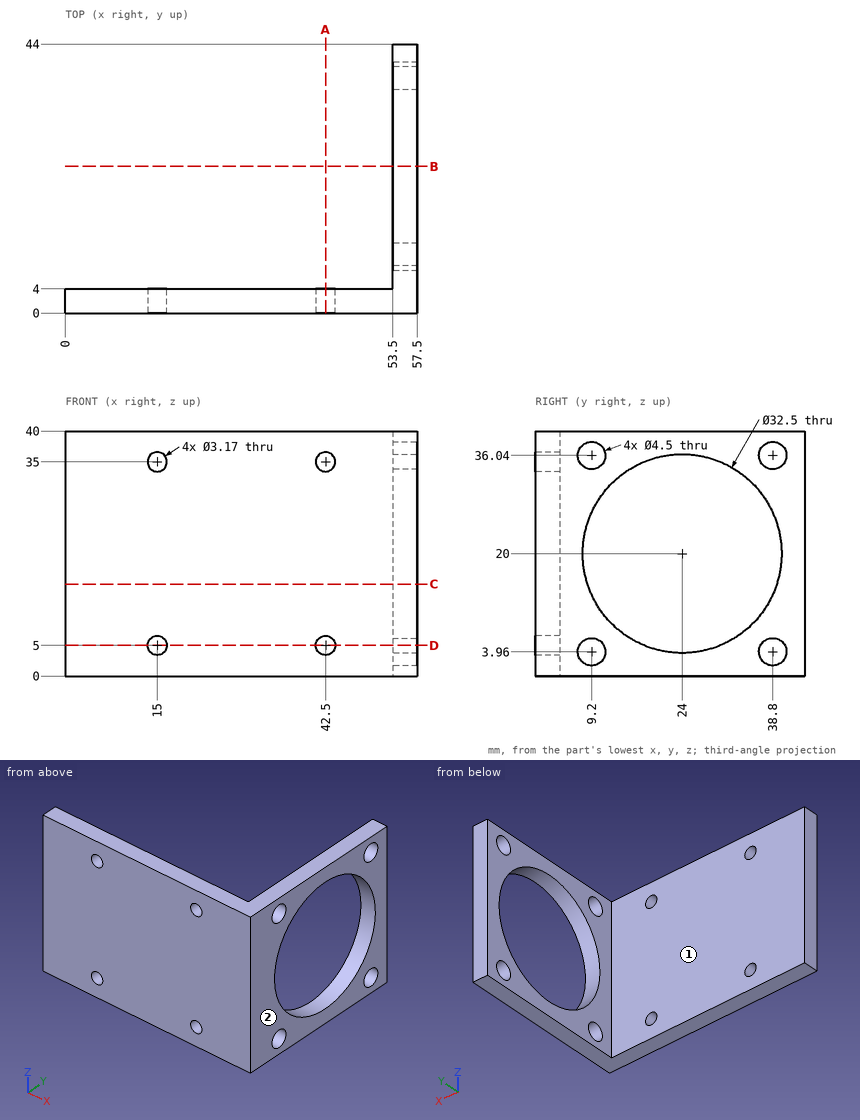
Print and shaded views of the part. All mm, measured from the part's lowest x, y and z. A direction names the side the tool comes from. Round coordinates to 2 decimals unless told otherwise and drop trailing zeros. Write each loop counter-clockwise with the first axis right and the second up, starting at its lowest first coordinate (ties: lowest second). Pieces come first, ordered by that corner, then holes. Notation, with made-up numbers: (-1, -10.5) -> (39, -10.5) arc R15 cw to (39, 1.5) -> close; hole circle Ø8 at (13, 17). An arc over 180 degrees is marked (long way). Answer in a Markdown table with one row per item. Add a question column.
Item 1: Which spindle directions (+Z, -Z, +X, -X, +Y, -Y) get a long thin tool onto all of the face, cutting with end or side? Do the marked faces 1 and 2. Say none if no direction does.
Item 2: Saw through at B-B, the plane y = 24. Write the cut outline in (x, z).
Item 3: Saw through at D-D, the plane z = 5. Write the cut outline in (x, y) (3 decimals), then the cut area to 3 significant figures.
Item 4: Drop flat-ended pins along their axis: pin 1 Ø12 at (x, z) = (17.5, 4) entering from +Y; pin 2 Ø5 at (y, z) = (9.2, 3.96) entering from -X. Give the stop position or say it passes through.
Item 5: Drill centre lines: line 1 (Z direction, x = 15, y = 3) (3 decimals); line 2 (X direction, y = 2.7, z = 5) (3 decimals); line 3 (Y direction, x = 54.5, z = 20). Where is each one in solid material? Low to high. Write a range as from..to.
Item 6: Saw through at A-A, the plane x = 42.5. Write the cut outline in (y, z) (3 decimals).
Item 7: Saw through at C-C, the plane z = 15. Write the cut outline in (x, y).
Findings below:
| question | item | result |
|---|---|---|
| 1 | face 1 | +Z, -Z, -X, +Y |
| 1 | face 2 | +Z, -Z, +X, +Y, -Y |
| 2 | outline | (53.5, 0) -> (57.5, 0) -> (57.5, 3.75) -> (53.5, 3.75) -> close; (53.5, 36.25) -> (57.5, 36.25) -> (57.5, 40) -> (53.5, 40) -> close |
| 3 | outline | (0, 0) -> (13.415, 0) -> (13.415, 4) -> (0, 4) -> close; (16.585, 0) -> (40.915, 0) -> (40.915, 4) -> (16.585, 4) -> close; (44.085, 0) -> (57.5, 0) -> (57.5, 7.205) -> (53.5, 7.205) -> (53.5, 4) -> (44.085, 4) -> close; (53.5, 11.195) -> (57.5, 11.195) -> (57.5, 17.75) -> (53.5, 17.75) -> close; (53.5, 30.25) -> (57.5, 30.25) -> (57.5, 36.805) -> (53.5, 36.805) -> close; (53.5, 40.795) -> (57.5, 40.795) -> (57.5, 44) -> (53.5, 44) -> close |
| 3 | area | 283 mm^2 |
| 4 | pin 1 | stops at y = 4 |
| 4 | pin 2 | stops at x = 53.5 |
| 5 | line 1 | z = 0..3.415, 6.585..33.415, 36.585..40 |
| 5 | line 2 | x = 0..13.415, 16.585..40.915, 44.085..57.5 |
| 5 | line 3 | y = 0..7.75, 40.25..44 |
| 6 | outline | (0, 0) -> (4, 0) -> (4, 3.415) -> (0, 3.415) -> close; (0, 6.585) -> (4, 6.585) -> (4, 33.415) -> (0, 33.415) -> close; (0, 36.585) -> (4, 36.585) -> (4, 40) -> (0, 40) -> close |
| 7 | outline | (0, 0) -> (57.5, 0) -> (57.5, 8.54) -> (53.5, 8.54) -> (53.5, 4) -> (0, 4) -> close; (53.5, 39.46) -> (57.5, 39.46) -> (57.5, 44) -> (53.5, 44) -> close |
